Work out the finished part from the listing and answer in its coordinate system (mm). A direction names the side the tool comes from. Coordinates: 2 decimals unless noted, no trailing zeros. Write each loop counter-clockwise with the first axis right and the second up, starting at its lowest first coordinate (ties: lowest second). Pieces come first, ordered by that corner, then holes. Notation, with made-up numbers: (30, -14.5) - (34, -14.5) arc R28 ccw to (34, 11.5) - close; hole circle Ø6 at (39, 1.5). An arc over 180 degrees is marked (long way). Answer as a JSON object with one key per item and string values. Group by question number.
from build123d import *

# Parameters (mm, degrees)
ESTRUSIONE_ESTRUSIONE1_DEPTH      = 45
ESTRUSIONE_ESTRUSIONE1_DEPTH_BACK = 3
SCHIZZO1_W                        = 25
SCHIZZO1_H                        = 2
SCHIZZO2_W                        = 42
SCHIZZO2_H                        = 2
ESTRUSIONE_ESTRUSIONE2_DEPTH      = 5


with BuildPart() as part:
    # Schizzo1 → Estrusione-Estrusione1 (new, two sides: drawn at the far end of the back side and taken through both)
    with BuildSketch(Plane.XY.offset(-ESTRUSIONE_ESTRUSIONE1_DEPTH_BACK)):
        with Locations((35.5, -54.5)):
            Rectangle(SCHIZZO1_W, SCHIZZO1_H)
    extrude(amount=ESTRUSIONE_ESTRUSIONE1_DEPTH + ESTRUSIONE_ESTRUSIONE1_DEPTH_BACK)

    # Schizzo2 → Estrusione-Estrusione2 (add)
    with BuildSketch(Plane(origin=(48, 0, 0), x_dir=(0, 0, -1), z_dir=(1, 0, 0))):
        with Locations((-21, -54.5)):
            Rectangle(SCHIZZO2_W, SCHIZZO2_H)
    estrusione_estrusione2 = extrude(amount=ESTRUSIONE_ESTRUSIONE2_DEPTH)

    # Specchia1: Estrusione-Estrusione2 across plane
    add(estrusione_estrusione2.mirror(Plane(origin=(35.5, 0, 0), x_dir=(0, 0, 1), z_dir=(1, 0, 0))))


solid = part.part
Q1. A tool of negligible diameter and unlimited length cuts with its end or side. For faces 1 (the face through (23, -55, -2)), 2 (the face through (48, -55, 43)), 3 (the face through (23, -55, 43)), from which of +Z, -Z, +X, -X, +Y, -Y can it reach the whole face along a straight path? Write none if from no direction.
Q2. Flat-ended cylindrical pins translate along their axes: pin 1 Ø0.6 at (y, z) = (-54.5, -2) entering from -X; pin 2 Ø0.6 at (y, z) = (-54.5, 43) entering from +X. Find the tip coordinate at first contact, or state that the pin passes through.
Q3. Consider L1, parallel to X at y = -53.8, z = -1; L2, parallel to Z at x = 49, y = -55.05. Determine where each line is inside the solid, lowest interval first. Write a range as from..to.
Q4. Section A-A on y = -54.8 is taken. Determine the outline of the cut face in (x, z), plus the area to 3 significant figures.
Q5. Section B-B on x = 50 is taken. Determine the outline of the cut face in (y, z).
Numbers:
{
 "1": {"face 1": "-Z, -X, +Y, -Y", "face 2": "+Z, +X, +Y, -Y", "face 3": "+Z, -X, +Y, -Y"},
 "2": {"pin 1": "stops at x = 23", "pin 2": "stops at x = 48"},
 "3": {"L1": "x = 23..48", "L2": "z = 0..42"},
 "4": {"outline": "(18, 0) - (23, 0) - (23, -3) - (48, -3) - (48, 0) - (53, 0) - (53, 42) - (48, 42) - (48, 45) - (23, 45) - (23, 42) - (18, 42) - close", "area": "1,620 mm²"},
 "5": {"outline": "(-55.5, 0) - (-53.5, 0) - (-53.5, 42) - (-55.5, 42) - close"}
}
